Autodesk Inventor part; units mm, degrees
ref_plane "Work Plane1" through (29, 0, 0) normal (0, -1, 0) x (1, 0, 0)
ref_plane "YZ Plane" through (0, 0, 0) normal (1, 0, 0) x (0, 1, 0)
ref_plane "XZ Plane" through (0, 0, 0) normal (0, 1, 0) x (-1, 0, 0)
sketch "Sketch1" plane through (0, 0, 0) normal (0, 0, 1) x (1, 0, 0)
  line L0 (-0.19, 0) -> (8, 0)
  line L1 (8, 0) -> (8, 2.5)
  line L2 (8, 2.5) -> (2.4, 2.5)
  line L3 (2.4, 2.5) -> (1.9091, 2.5)
  line L4 (1.9091, 2.5) -> (0, 2.5)
  line L5 (0, 2.5) -> (0, 4.75)
  line L6 (0, 4.75) -> (-2.75, 4.75)
  line L7 (-2.75, 4.75) -> (-2.75, 1.7321)
  line L8 (-2.75, 1.7321) -> (-1.19, 1.7321)
  line L9 (-1.19, 1.7321) -> (-0.19, 0)
  line L10 (-4.9, 0) -> (10.15, 0)
  line L11 (0, -0.95) -> (0, 5.7)
  line L12 (2.4, 2.5) -> (0, 2.5) construction
  dimension "d1" = 5.6
  dimension "d2" = 0.4909
  dimension "d3" = 2.75
  dimension "d4" = 1.56
  dimension "d5" = 60
  dimension "d6" = 5
  dimension "d7" = 5
  dimension "d8" = 3.4641
  dimension "d9" = 9.5
  dimension "d26" = 8
revolve "Body" add sketch "Sketch1" angle 360 about axis through (-0.19, 0, 0) along (1, 0, 0)
sketch "Sketch2" plane through (-2.75, 0, 0) normal (-1, 0, 0) x (0, 0, 1)
  circle A0 centre (0, 0) radius 1.7321
  line L0 (0, -6.65) -> (0, 6.65)
  line L1 (-6.65, 0) -> (6.65, 0)
  line L2 (1.7321, 0) -> (0.866, -1.5)
  line L3 (0.866, -1.5) -> (-0.866, -1.5)
  line L4 (-0.866, -1.5) -> (-1.7321, 0)
  line L5 (-1.7321, 0) -> (-0.866, 1.5)
  line L6 (-0.866, 1.5) -> (0.866, 1.5)
  line L7 (0.866, 1.5) -> (1.7321, 0)
extrude "Slot" add sketch "Sketch2" against normal up to next contours L7 A0 | A0 L2 | L6 L0 A0 | A0 L0 L3 | L0 L6 A0 | A0 L3 L0 | L4 A0 | A0 L5
fillet "Fillet1" radius 2.37 1 edges at (-2.75, -4.75, 0)
thread "Thread"
chamfer "Chamfer1" distance 0.4908 distance2 0.4908 1 edges at (8, -2.5, 0) measured on face at (8, -0.6238, -0.819)
ref_plane "Work Plane1" through (29, 0, 0) normal (0, -1, 0) x (1, 0, 0)
fillet "Fillet2" radius 0.45 1 edges at (0, -2.5, 0)
equation "\"d30\" = R"
equation "\"d17\" = RR"
equation "\"d13\" = GEL"
equation "\"d15\" = -0.5 * SPD + 0.5 * GD"
equation "\"d16\" = GUL"
equation "\"d1\" = GEL"
equation "\"d3\" = KOH"
equation "\"d4\" = INTI"
equation "\"d6\" = GD"
equation "\"d7\" = BDM"
equation "\"d8\" = 1.1547 * SW"
equation "\"d9\" = KOD"
equation "\"d26\" = NLG"
equation "\"GD\" = NND"
equation "\"NLG\" = 8"
equation "\"GEL\" = 5.6"
equation "\"KOD\" = 9.5"
equation "\"KOH\" = 2.75"
equation "\"INTI\" = 1.56"
equation "\"GAL\" = 0.61345 * PTC"
equation "\"GUL\" = 0.61345 * PTC"
equation "\"BDM\" = NND"
equation "\"SW\" = 3"
equation "\"RR\" = 2.37"
equation "\"SPD\" = NND - 1.2269 * PTC"
equation "\"R\" = 0.45"
equation "\"TOA\" = 30deg"
equation "\"GD1\" = THREADDIA - 1.2269 * PTC"
equation "\"THREADDIA\" = 5"
equation "\"PTC\" = 0.8"
equation "\"NND\" = 5"
equation "\"KOH1\" = 0.38"
equation "\"E0\" = 3.443"
properties part number "ISO 7380-1 - M5 x 8" material "Steel"
Here's how the part is built. I have some questions about the finished solid (model axes, mm). A direction names the side the tool comes from. Round coordinates to 2 decimals unless told otherwise and drop trailing zeros. Loops run counter-clockwise (first coordinate to the right, second up) from the corner with the lowest first, then second, coordinate; pieces in that order, holes last.
1. If we section it at B-B on x = 1.25: Write out the boundary of the cut face in (y, z), plus the area to 3 significant figures.
Answer list:
outline: circle Ø5 at (0, 0)
area: 19.6 mm2
2. Which directions (+Z, -Z, +X, -X, +Y, -Y) give clear straight access to the entire face, cutting with the end or side of a thin tool? Please do faces 1 (the face through (8, 0, 0)), 2 (the face through (3.93, -0.54, 2.44)), 3 (the face through (-2, -1.5, 0)).
Answer list:
face 1: +Z, -Z, +X, +Y, -Y
face 2: +X
face 3: -X
3. If I drill on line 1 along Z through (x, y) = (-1.5, -1.25); line 2 along Z through (x, y) = (1, 0); line 3 along Z through (x, y) = (-0.75, -0.5), over which ranges is the centre line in solid material (lowest first)?
Answer list:
line 1: z = -4.29 to -1.01, 1.01 to 4.29
line 2: z = -2.5 to 2.5
line 3: z = -4.69 to -0.83, 0.83 to 4.69
4. For P1, Ø3, axis at x = 4, y = 1, coming from the -Z side; P2, Ø1.5, axis at x = -0.5, z = -3, coming from the -Y side; P3, Ø1.5, axis at x = 6, y = -3, coming from the +Z side, each with a flat end and sliding along its axis, tell me the tip position at first contact or that it passes through.
Answer list:
P1: stops at z = -2.5
P2: stops at y = -4.18
P3: stops at z = 1.09
5. If we section it at A-A on x = -2: Write out the boundary of the cut face in (y, z).
Answer list:
outline: circle Ø8.22 at (0, 0); hole (-1.5, -0.87) - (0, -1.73) - (1.5, -0.87) - (1.5, 0.87) - (0, 1.73) - (-1.5, 0.87) - close
6. We'd pull the mould along Y, two halves only. Please class faces 4 (the face through (-1.915, -0.761, -1.293)), 5 (the face through (-0.193, 2.192, 4.214)), 6 (the face through (0, -0.1, -3.1)), 7 (the face through (-2, 1.5, 0)): +Y half, -Y half, draft (parallel to the pull), parting line (faces both ways), or undercut.
Answer list:
face 4: undercut
face 5: parting line
face 6: draft
face 7: undercut
